from build123d import *

# Parameters (mm, degrees)
CYLINDER_R        = 3.3
CYLINDER_DEPTH    = 20
CYLINDER001_R     = 3.3
CYLINDER001_DEPTH = 20
CYLINDER002_R     = 3.3
CYLINDER002_DEPTH = 20
CYLINDER003_R     = 6
CYLINDER003_DEPTH = 19
CYLINDER004_R     = 6
CYLINDER004_DEPTH = 19
CYLINDER005_R     = 6
CYLINDER005_DEPTH = 19
BOX_W             = 20
BOX_H             = 20
BOX_DEPTH         = 20
FILLET_R          = 1.5


with BuildPart() as cylinder:
    # Cylinder → Cylinder (new body)
    with BuildSketch(Plane(origin=(10, 10, 0), x_dir=(1, 0, 0), z_dir=(0, 0, 1))):
        Circle(CYLINDER_R)
    extrude(amount=CYLINDER_DEPTH)


with BuildPart() as cylinder001:
    # Cylinder001 → Cylinder001 (new body)
    with BuildSketch(Plane(origin=(10, 20, 10), x_dir=(1, 0, 0), z_dir=(0, -1, 0))):
        Circle(CYLINDER001_R)
    extrude(amount=CYLINDER001_DEPTH)


with BuildPart() as cylinder002:
    # Cylinder002 → Cylinder002 (new body)
    with BuildSketch(Plane(origin=(0, 10, 10), x_dir=(0, 0, -1), z_dir=(1, 0, 0))):
        Circle(CYLINDER002_R)
    extrude(amount=CYLINDER002_DEPTH)


with BuildPart() as cylinder003:
    # Cylinder003 → Cylinder003 (new body)
    with BuildSketch(Plane(origin=(0, 10, 10), x_dir=(0, 0, -1), z_dir=(1, 0, 0))):
        Circle(CYLINDER003_R)
    extrude(amount=CYLINDER003_DEPTH)


with BuildPart() as cylinder004:
    # Cylinder004 → Cylinder004 (new body)
    with BuildSketch(Plane(origin=(10, 10, 0), x_dir=(1, 0, 0), z_dir=(0, 0, 1))):
        Circle(CYLINDER004_R)
    extrude(amount=CYLINDER004_DEPTH)


with BuildPart() as fusion:
    # Cylinder005 → Cylinder005 (new body)
    with BuildSketch(Plane(origin=(10, 20, 10), x_dir=(1, 0, 0), z_dir=(0, -1, 0))):
        Circle(CYLINDER005_R)
    extrude(amount=CYLINDER005_DEPTH)

    # Fusion: union Cylinder, Cylinder001, Cylinder002, Cylinder003, Cylinder004
    add(cylinder.part)
    add(cylinder001.part)
    add(cylinder002.part)
    add(cylinder003.part)
    add(cylinder004.part)


with BuildPart() as f_20x20connectorcube:
    # Box → Box (new body)
    with BuildSketch(Plane.XY):
        with Locations((10, 10)):
            Rectangle(BOX_W, BOX_H)
    extrude(amount=BOX_DEPTH)

    # Cut: cut Fusion
    add(fusion.part, mode=Mode.SUBTRACT)

    # Fillet
    fillet_edges = [f_20x20connectorcube.edges().sort_by_distance(p)[0] for p in [
        (0, 10, 0),
        (0, 20, 10),
        (10, 20, 0),
    ]]
    fillet(fillet_edges, radius=FILLET_R)


solid = f_20x20connectorcube.part
Here's how the part is built. I have some questions about the finished solid (model axes, mm). A direction names the side the tool comes from. Give positions to 0.01 mm unless a question says otherwise; leave off trailing zeros. Order: outer loops, then holes, each group sorted by start corner. A loop starts at its lowest first (then second) coordinate and runs counter-clockwise, first axis right, second up. Notation, with made-up numbers: (68.5, -4.5) -> (107.5, -4.5) arc R22 cw to (107.5, 15.5) -> close; hole circle Ø11 at (25, 50). An arc over 180 degrees is marked (long way). One line per item, written item: value. Start each with the question number.
1. We'd pull the mould along Z, two halves only. Please class faces 4 (the face through (15, 5, 0)), 5 (the face through (20, 10, 5)), 6 (the face through (13, 1, 7)), 7 (the face through (7.381, 0.507, 7.992)): released by +Z, released by -Z, zero draft, split by the parting line, or undercut.
2. Imagine slicing it at C-C, the plane x = 15.5. List the corners of the cut face in (y, z) for me, plus the area to 3 significant figures.
3. Imagine slicing it at A-A, the plane z = 10. List the corners of the cut face in (x, y) for me, plus the area to 3 significant figures.
4. Imagine slicing it at D-D, the plane y = 5.25. List the corners of the cut face in (x, z) for me.
5. Will these pins go through, and if not, where does the flat tip stop? pin 1 Ø3.5 at (y, z) = (7.5, 8.5) entering from -X; pin 2 Ø1.5 at (x, y) = (8.5, 14.5) entering from -Z; pin 3 Ø4 at (x, z) = (10, 10) entering from -Y.
6. Imagine slicing it at B-B, the plane y = 10. List the corners of the cut face in (x, z) for me.
7. I need wall thicknesses on probe 1 along X at (y, z) = (10, 19.75); probe 2 along Y at (x, z) = (10, 16.2). Which ranges of each line are inside material? Lowest first, please. Write a range as from..to.
8. For faces 1 (the face through (19, 7, 7)), 2 (the face through (5.58, 14.06, 2.2)), 3 (the face through (4, 3, 10)), which set-ups out of +Z, -Z, +X, -X, +Y, -Y let a thin tool reach every point of the face, with its end or its side?
Values follow:
1. face 4: released by -Z
1. face 5: zero draft
1. face 6: undercut
1. face 7: undercut
2. outline: (0, 0) -> (7.6, 0) -> (7.6, 4.5) arc R6 cw to (4.5, 7.6) -> (1, 7.6) -> (1, 12.4) -> (4.5, 12.4) arc R6 cw to (7.6, 15.5) -> (7.6, 19) -> (12.4, 19) -> (12.4, 15.5) arc R6 cw to (15.5, 12.4) -> (20, 12.4) -> (20, 20) -> (0, 20) -> close; (12.4, 0) -> (18.5, 0) arc R1.5 ccw to (20, 1.5) -> (20, 7.6) -> (15.5, 7.6) arc R6 cw to (12.4, 4.5) -> close
2. area: 216 mm2
3. outline: (0, 0) -> (6.7, 0) -> (6.7, 1) -> (4, 1) -> (4, 4) -> (0, 4) -> close; (0, 16) -> (4, 16) -> (4, 20) -> (1.5, 20) arc R1.5 ccw to (0, 18.5) -> close; (13.3, 0) -> (20, 0) -> (20, 6.7) -> (19, 6.7) -> (19, 4) -> (16, 4) -> (16, 1) -> (13.3, 1) -> close; (16, 16) -> (19, 16) -> (19, 13.3) -> (20, 13.3) -> (20, 20) -> (16, 20) -> close
3. area: 74.3 mm2
4. outline: (0, 1.5) arc R1.5 ccw to (1.5, 0) -> (6.33, 0) -> (6.33, 5.25) arc R6 cw to (5.25, 6.33) -> (0, 6.33) -> close; (0, 13.67) -> (5.25, 13.67) arc R6 cw to (6.33, 14.75) -> (6.33, 19) -> (13.67, 19) -> (13.67, 14.75) arc R6 cw to (14.75, 13.67) -> (19, 13.67) -> (19, 6.33) -> (14.75, 6.33) arc R6 cw to (13.67, 5.25) -> (13.67, 0) -> (20, 0) -> (20, 20) -> (0, 20) -> close
5. pin 1: stops at x = 19
5. pin 2: stops at z = 19
5. pin 3: passes through
6. outline: (0, 1.5) arc R1.5 ccw to (1.5, 0) -> (4, 0) -> (4, 4) -> (0, 4) -> close; (0, 16) -> (4, 16) -> (4, 19) -> (6.7, 19) -> (6.7, 20) -> (0, 20) -> close; (13.3, 19) -> (16, 19) -> (16, 16) -> (19, 16) -> (19, 13.3) -> (20, 13.3) -> (20, 20) -> (13.3, 20) -> close; (16, 0) -> (20, 0) -> (20, 6.7) -> (19, 6.7) -> (19, 4) -> (16, 4) -> close
7. probe 1: x = 0..6.7, 13.3..20
7. probe 2: y = 0..4, 16..20
8. face 1: -X
8. face 2: -Z
8. face 3: +Y
